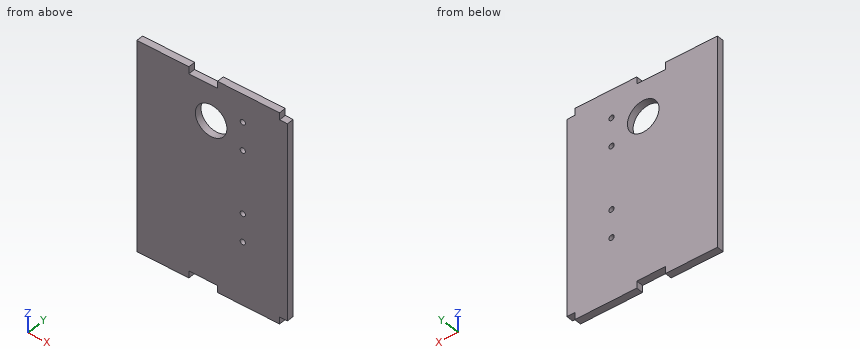
```python
from build123d import *

# Parameters (mm, degrees)
SKETCH1_W           = 304.8
SKETCH1_H           = 355.6
SKETCH1_RX          = 28.575
SKETCH1_RY          = 28.573991153
BOSS_EXTRUDE1_DEPTH = 12.7
SKETCH2_R           = 4.7625
CUT_EXTRUDE1_DEPTH  = 12.7
SKETCH3_W           = 112.268
SKETCH3_H           = 12.7
BOSS_EXTRUDE2_DEPTH = 12.7
SKETCH5_W           = 38.383719954
SKETCH5_H           = 381
CUT_EXTRUDE2_DEPTH  = 13.7


with BuildPart() as part:
    # Sketch1 → Boss-Extrude1 (new body)
    with BuildSketch(Plane(origin=(0, 0, 0), x_dir=(1, 0, 0), z_dir=(0, 1, 0))):
        with Locations((152.4, 177.8)):
            Rectangle(SKETCH1_W, SKETCH1_H)
        with Locations(Location((166.724174942, 64.195003676), (0, 0, 0))):
            Ellipse(SKETCH1_RX, SKETCH1_RY, mode=Mode.SUBTRACT)
    extrude(amount=BOSS_EXTRUDE1_DEPTH)

    # Sketch2 → Cut-Extrude1 (cut)
    with BuildSketch(Plane.XZ):
        with Locations((224.028, -38.1)):
            Circle(SKETCH2_R)
        with Locations((224.028, -88.9)):
            Circle(SKETCH2_R)
        with Locations((224.028, -203.2)):
            Circle(SKETCH2_R)
        with Locations((224.028, -254)):
            Circle(SKETCH2_R)
    extrude(amount=-CUT_EXTRUDE1_DEPTH, mode=Mode.SUBTRACT)

    # Sketch3 → Boss-Extrude2 (add)
    with BuildSketch(Plane(origin=(0, 12.7, 0), x_dir=(1, 0, 0), z_dir=(0, 1, 0))):
        with Locations((70.358, 361.95)):
            Rectangle(SKETCH3_W, SKETCH3_H)
        with Locations((234.442, 361.95)):
            Rectangle(SKETCH3_W, SKETCH3_H)
        with Locations((234.442, -6.35)):
            Rectangle(SKETCH3_W, SKETCH3_H)
        with Locations((70.358, -6.35)):
            Rectangle(SKETCH3_W, SKETCH3_H)
    extrude(amount=-BOSS_EXTRUDE2_DEPTH)

    # Sketch5 → Cut-Extrude2 (cut, through all)
    with BuildSketch(Plane.XZ):
        with Locations((13.259015168, -177.8)):
            Rectangle(SKETCH5_W, SKETCH5_H)
    extrude(amount=-CUT_EXTRUDE2_DEPTH, mode=Mode.SUBTRACT)


solid = part.part
```
The model under review builds one solid part; all positions refer to its coordinate system, in mm. Round coordinates to 2 decimals unless told otherwise and drop trailing zeros. Write each loop counter-clockwise with the first axis right and the second up, starting at its lowest first coordinate (ties: lowest second). Pieces come first, ordered by that corner, then holes.
(1) Insertion check: pin 1 (6.5 mm diameter, centred on x = 300.5, y = 6.5, fed in from +Z); pin 2 (8.5 mm diameter, centred on x = 224.028, z = -88.9, fed in from +Y); pin 3 (11 mm diameter, centred on x = 224.028, z = -254, fed in from -Y). Each pin has a flat end and moves straight along its axis. Give the tip position at first contact, or say it passes through.
(2) We need section B-B on z = -88.9. Give the number of separate pieces and of enclosed holes in the cut face, and give its area (3 significant figures).
(3) We need section A-A on z = -203.2. Give the boundary of the cut face in (x, y).
(4) Wall thickness on L1, parallel to Z at x = 165, y = 6.75; L2, parallel to X at y = 7.75, z = -52: over which ranges is each line inside the solid? List them lowest first.
Findings below:
1. pin 1: stops at z = 0
1. pin 2: passes through
1. pin 3: stops at y = 0
2. separate pieces: 3
2. enclosed holes: 0
2. area: 2,970 mm2
3. outline: (32.45, 0) - (219.27, 0) - (219.27, 12.7) - (32.45, 12.7) - close; (228.79, 0) - (304.8, 0) - (304.8, 12.7) - (228.79, 12.7) - close
4. L1: z = -355.6 to -92.72, -35.67 to 0
4. L2: x = 32.45 to 140.88, 192.57 to 304.8
